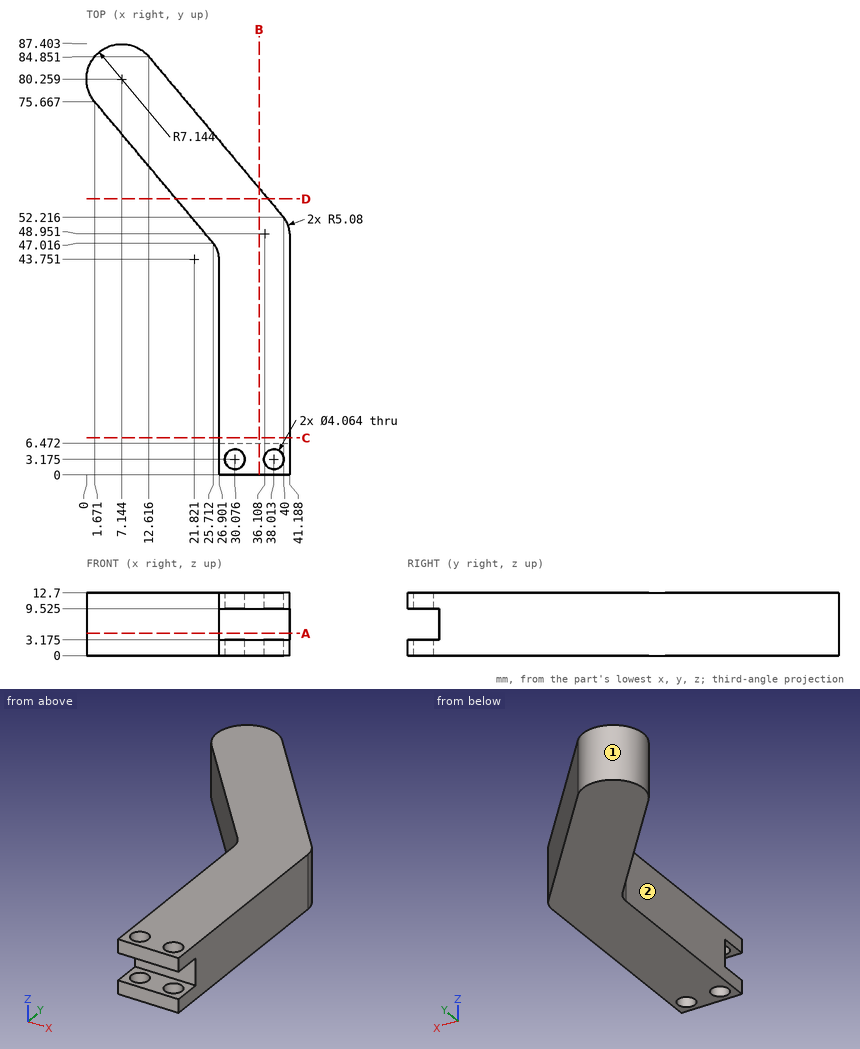
Verification items for this drawing (mm, ordinates from the low corner). A direction names the side the tool comes from. Round coordinates to 2 decimals unless told otherwise and drop trailing zeros. Order: outer loops, then holes, each group sorted by start corner. A loop starts at its lowest first (then second) coordinate and runs counter-clockwise, first axis right, second up. Notation, with made-up numbers: M -13,-31 L 40,-31 A23 cw 40,-5 Z; hole C -40,9 d6. An arc over 180 degrees is marked long. Answer in a Markdown table with one row per item. Add a question column.
Item 1: Sectioned sample at B-B, the plane x = 35. Enter the section's corners in (y, z) (1 decimal), plus the area to 3 significant figures.
Item 2: Material ranges on L1, parallel to X at y = 12, z = 0.5; L2, parallel to X at y = 55.5, z = 11 (1 decimal); L3, parallel to Y at x = 10, z = 6.75 (1 decimal), recorded low to high. Write a range as [from, to].
Item 3: Sectioned sample at D-D, the plane y = 56. Enter the section's corners in (x, z) (1 decimal).
Item 4: Depth check by flat-ended pin: pin 1 Ø1 at (x, z) = (10, 10) entering from -Y (1 decimal); pin 2 Ø5 at (x, y) = (37.5, 1.5) entering from +Z; pin 3 Ø5 at (x, z) = (4.5, 6) entering from -Y (1 decimal); pin 4 Ø4 at (y, z) = (70.5, 7.5) entering from +X (1 decimal). Enter the tip coordinate at first touch or a pass-through.
Item 5: Sectioned sample at C-C, the plane y = 7.5. Enter the section's corners in (x, z).
Item 6: Sectioned sample at A-A, the plane z = 4.5. Enter the section's corners in (x, y), plus the area to 3 significant figures.
Item 7: Set-up check for the marked faces 1 and 2: record each of +Z, -Z, +X, -X, +Y, -Y from which the full face is reachable in a straight line by a thin tool's end or side.
Filled in:
| question | item | result |
|---|---|---|
| 1 | outline | M 0,0 L 58.2,0 L 58.2,12.7 L 0,12.7 L 0,9.5 L 6.5,9.5 L 6.5,3.2 L 0,3.2 Z |
| 1 | area | 698 mm² |
| 2 | L1 | x = [26.9, 41.19] |
| 2 | L2 | x = [18.6, 37.2] |
| 2 | L3 | y = [65.7, 86.8] |
| 3 | outline | M 18.2,0 L 36.8,0 L 36.8,12.7 L 18.2,12.7 Z |
| 4 | pin 1 | stops at y = 65.1 |
| 4 | pin 2 | stops at z = 12.7 |
| 4 | pin 3 | stops at y = 69.3 |
| 4 | pin 4 | stops at x = 26.3 |
| 5 | outline | M 26.9,0 L 41.19,0 L 41.19,12.7 L 26.9,12.7 Z |
| 6 | outline | M 1.67,75.67 L 25.71,47.02 A5.08 cw 26.9,43.75 L 26.9,6.47 L 41.19,6.47 L 41.19,48.95 A5.08 ccw 40,52.22 L 12.62,84.85 A7.14 ccw Z |
| 6 | area | 1,270 mm² |
| 7 | face 1 | +Z, -Z |
| 7 | face 2 | +Z, -Z, -X, -Y |
